```python
from build123d import *

# Parameters (mm, degrees)
SZKIC1_R                        = 19
DODANIE_WYCI_GNI_CIE1_DEPTH     = 8.3
WYTNIJ_WYCI_GNI_CIE1_DEPTH      = 1036.988363246
WYTNIJ_WYCI_GNI_CIE1_DEPTH_BACK = 1036.988363246
SZKIC2_R                        = 3
WYTNIJ_WYCI_GNI_CIE2_START      = 8.3
SZKIC3_R                        = 5.5
WYTNIJ_WYCI_GNI_CIE2_DEPTH      = 6.3


with BuildPart() as part:
    # Szkic1 → Dodanie-wyciągnięcie1 (new body)
    with BuildSketch(Plane(origin=(0, 0, 0), x_dir=(1, 0, 0), z_dir=(0, 1, 0))):
        with Locations(Location((0, 0, 0), (0, 0, 90))):
            Circle(SZKIC1_R)
    extrude(amount=DODANIE_WYCI_GNI_CIE1_DEPTH)

    # Szkic2 → Wytnij-wyciągnięcie1 (cut, two sides: drawn at the far end of the back side and taken through both)
    with BuildSketch(Plane(origin=(141.849854944, -17.369665232, -1004.103260298), x_dir=(0.9996501322683511, 0, -0.02645019954306737), z_dir=(0, 1, 0)).offset(-WYTNIJ_WYCI_GNI_CIE1_DEPTH_BACK)):
        with Locations(Location((-181.587823501, -1000, 0), (0, 0, 268.484338434))):
            Circle(SZKIC2_R)
        with Locations(Location((-166.587823501, -1000, 0), (0, 0, 268.484338434))):
            Circle(SZKIC2_R)
    extrude(amount=WYTNIJ_WYCI_GNI_CIE1_DEPTH + WYTNIJ_WYCI_GNI_CIE1_DEPTH_BACK, mode=Mode.SUBTRACT)

    # Szkic3 → Wytnij-wyciągnięcie2 (cut)
    with BuildSketch(Plane(origin=(0, 0, 0), x_dir=(1, 0, 0), z_dir=(0, 1, 0)).offset(WYTNIJ_WYCI_GNI_CIE2_START)):
        with Locations(Location((-13.224237294, -0.349906136, 0), (0, 0, 270))):
            Circle(SZKIC3_R)
        with Locations(Location((1.77051469, 0.046846857, 0), (0, 0, 270))):
            Circle(SZKIC3_R)
    extrude(amount=-WYTNIJ_WYCI_GNI_CIE2_DEPTH, mode=Mode.SUBTRACT)


solid = part.part
```
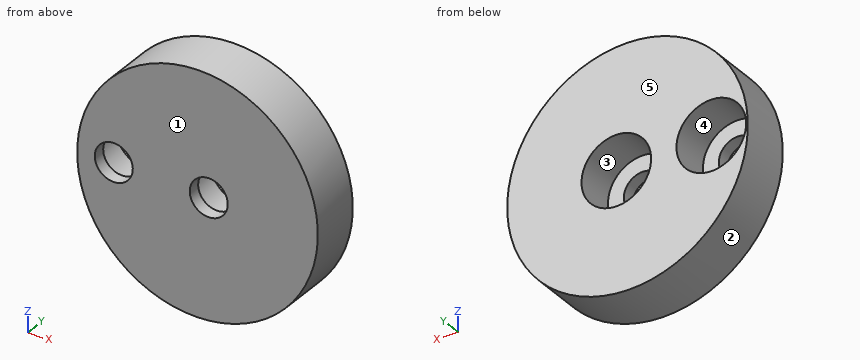
Input: part model. Units: mm. Frame: model coordinates. Face numbers are marked on the shaded views. A direction names the side the tool comes from. Round coordinates to 2 decimals unless told otherwise and drop trailing zeros. Write each loop counter-clockwise with the first axis right and the second up, starting at its lowest first coordinate (ties: lowest second). Pieces come first, ordered by that corner, then holes. Notation, with made-up numbers: (62.25, 27.5) - (110.25, 27.5) arc R19 ccw to (110.25, 43.5) - close; hole circle Ø7 at (6, 77). An arc over 180 degrees is marked (long way). Write item = value, one per line.
(1) Section query D-D on y = 6.75. Output: boundary loops of the cut face in (x, z).
Geometry check:
outline = circle Ø38 at (0, 0); hole circle Ø11 at (-13.22, 0.35); hole circle Ø11 at (1.77, -0.05)
(2) Access query for the marked faces 4 and 5. Directions: +Z, -Z, +X, -X, +Y, -Y. A direction counts if a zero-diameter tool reaches every point of the face in a straight line with its end or side. Return the directions, or none.
Geometry check:
face_4 = +Y
face_5 = +Z, -Z, +X, -X, +Y
(3) Material intervals for probe 1 along X at (y, z) = (6.25, -3); probe 2 along X at (y, z) = (3.5, 3); probe 3 along Z at (x, y) = (1.5, 2.5), sorted ascending.
Geometry check:
probe_1 = -18.76 to -17.59, -8.86 to -2.87, 6.41 to 18.76
probe_2 = -18.76 to -18.04, -8.4 to -2.81, 6.35 to 18.76
probe_3 = -18.94 to -5.54, 5.45 to 18.94
(4) Section query A-A on x = 0. Output: boundary loops of the cut face in (y, z), then the cut area to 3 significant figures.
Geometry check:
outline = (0, -19) - (8.3, -19) - (8.3, -5.25) - (2, -5.25) - (2, -2.47) - (0, -2.47) - close; (0, 2.37) - (2, 2.37) - (2, 5.16) - (8.3, 5.16) - (8.3, 19) - (0, 19) - close
area = 240 mm^2
(5) Pull-direction query (X, two-part tool) for the marked faces 1, 2 and 3; classes: +X half, -X half, draft (parallel to the pull), parting line (faces both ways), or undercut.
Geometry check:
face_1 = draft
face_2 = parting line
face_3 = undercut
(6) Section query B-B on z = 0. Output: boundary loops of the cut face in (x, y), then the cut area to 3 significant figures.
Geometry check:
outline = (-19, 0) - (-16.2, 0) - (-16.2, 2) - (-18.71, 2) - (-18.71, 8.3) - (-19, 8.3) - close; (-10.24, 0) - (-1.23, 0) - (-1.23, 2) - (-3.73, 2) - (-3.73, 8.3) - (-7.74, 8.3) - (-7.74, 2) - (-10.24, 2) - close; (4.77, 0) - (19, 0) - (19, 8.3) - (7.27, 8.3) - (7.27, 2) - (4.77, 2) - close
area = 153 mm^2
(7) Contact query for flat-ended pins moving along their axis: pin 1 Ø3.5 at (x, z) = (1.5, -1.5) entering from +Y; pin 2 Ø1 at (y, z) = (5.5, -11) entering from +X. Output: stop coordinate, or through.
Geometry check:
pin_1 = 2
pin_2 = 15.84
(8) Section query C-C on z = 5. Output: boundary loops of the cut face in (x, y), then the cut area to 3 significant figures.
Geometry check:
outline = (-18.33, 0) - (18.33, 0) - (18.33, 8.3) - (3.96, 8.3) - (3.96, 2) - (-0.42, 2) - (-0.42, 8.3) - (-10.29, 8.3) - (-10.29, 2) - (-16.16, 2) - (-16.16, 8.3) - (-18.33, 8.3) - close
area = 240 mm^2
